Part model, mm, in its own coordinate system. A direction names the side the tool comes from. Round coordinates to 2 decimals unless told otherwise and drop trailing zeros. Write each loop counter-clockwise with the first axis right and the second up, starting at its lowest first coordinate (ties: lowest second). Pieces come first, ordered by that corner, then holes. Notation, with made-up numbers: (14.5, -8.75) -> (34.5, -8.75) arc R22 ccw to (34.5, 12.25) -> close; hole circle Ø6 at (45, 28). An arc over 180 degrees is marked (long way). Use CSV: the item, a comma, the result in double quotes. Start each with the question number.
(1) Saw through at A-A (y = 13.5). Give the cut face in (x, z) (3 decimals).
(2) Saw through at D-D (y = 4.5). Give the cut face in (x, z), plus the area to 3 significant figures.
(3) Saw through at B-B (x = 0.25). Count the separate pieces of the cut face and the enclosed holes in it, plus the area to 3 significant figures.
(4) Saw through at C-C (z = 11.5). Give the cut face in (x, y) (3 decimals), plus the area to 3 significant figures.
(5) Probe line 1 (X direction, y = 1, z = 13) (3 decimals); line 2 (X direction, y = 9.5, z = 9.25); line 3 (Y direction, x = 7, z = 2.75). List the from-to ranges inside material, lowest first. Write a range as [from, to].
(6) Drop flat-ended pins along their axis: pin 1 (0.9 mm diameter, centred on y = -0.5, z = 16.5, fed in from -X); pin 2 (0.5 mm diameter, centred on y = 2.5, z = -0.5, fed in from +X); pin 3 (1.2 mm diameter, centred on x = 1, y = -0.5, fed in from -Z); pin 4 (9 mm diameter, centred on y = 10.5, z = 15.5, fed in from -X). Give the stop position or say it passes through.
(7) Which spindle directions (+Z, -Z, +X, -X, +Y, -Y) get a long thin tool onto all of the face, cutting with end or side? Do faces 5 (the flat face through (-2.315, 11, 1)), 6 (the flat face through (-2.86, -0.5, 16.7)), 7 (the flat face through (-2.315, 1, 11)), 8 (the flat face through (-5.92, 9, 9)), 9 (the flat face through (0, 16.18, -0.5)). Say none if no direction does.
(8) Two-plate mould, pull along Y, no slides. Class faces 1 (the flat face through (0, 2.1, -0.5)), 2 (the flat face through (0, 17.26, -0.5)), 3 (the flat face through (0, -0.5, 2.1)), 4 (the flat face through (0, 7.33, 1)): released by +Y, released by -Y, zero draft, split by the parting line, or undercut.
```python
from build123d import *

# Parameters (mm, degrees)
BOSS_EXTRUDE2_DEPTH     = 7.5
CAVITY_START            = 2
SKETCH3_W               = 5.92
SKETCH3_H               = 9.5
CAVITY_DEPTH            = 23.259018941
SLOT_CUT_REACH          = 26.259
SQUARE_START            = -2
SKETCH8_W               = 2.315
SKETCH8_H               = 6.67
SQUARE_SLOT_DEPTH       = 2
BOSS_EXTRUDE3_DEPTH     = 0.8
SKETCH9_W               = 2.86
SKETCH9_H               = 1.08
SQUARE_RAILS_DEPTH      = 1.08
HALF_START              = 5.92
HALF_MIRROR_DEPTH       = 1.58
HALF_MIRROR_2_OUTLINE_W = 6
HALF_MIRROR_2_OUTLINE_H = 2
HALF_MIRROR_2_DEPTH     = 5.92
HALF_START_2            = 2.315
HALF_MIRROR_3_OUTLINE_W = 6.67
HALF_MIRROR_3_OUTLINE_H = 2
HALF_MIRROR_3_DEPTH     = 3.605
HALF_MIRROR_4_OUTLINE_W = 1.08
HALF_MIRROR_4_OUTLINE_H = 1.08
HALF_MIRROR_4_DEPTH     = 2.86
FULL_START              = -7.5
FULL_MIRROR_OUTLINE_W   = 2
FULL_MIRROR_OUTLINE_H   = 6
FULL_MIRROR_DEPTH       = 15
FULL_MIRROR_2_DEPTH     = 1.58
FULL_START_2            = 5.92
FULL_MIRROR_3_DEPTH     = 1.58
FULL_START_3            = -5.92
FULL_MIRROR_4_OUTLINE_W = 2
FULL_MIRROR_4_OUTLINE_H = 6.67
FULL_MIRROR_4_DEPTH     = 3.605
FULL_START_4            = 2.315
FULL_MIRROR_5_OUTLINE_W = 2
FULL_MIRROR_5_OUTLINE_H = 6.67
FULL_MIRROR_5_DEPTH     = 3.605
FULL_START_5            = -2.86
FULL_MIRROR_6_OUTLINE_W = 1.08
FULL_MIRROR_6_OUTLINE_H = 1.08
FULL_MIRROR_6_DEPTH     = 5.72


# Read off the part's stored shape, not the designer's step: Half mirror, Full mirror
with BuildPart() as part:
    # Sketch2 → Boss-Extrude2 (new body)
    with BuildSketch(Plane(origin=(0, 0, 0), x_dir=(0, 0, -1), z_dir=(1, 0, 0))):
        Polygon((-11.5, 11.5), (-3, 20), (0, 20), (0, 0), align=None)
    extrude(amount=-BOSS_EXTRUDE2_DEPTH)

    # Sketch3 → Cavity (cut, through all)
    with BuildSketch(Plane(origin=(0, 0, 0), x_dir=(1, 0, 0), z_dir=(0, 1, 0)).offset(CAVITY_START)):
        with Locations((-2.96, -6.75)):
            Rectangle(SKETCH3_W, SKETCH3_H)
    extrude(amount=CAVITY_DEPTH, mode=Mode.SUBTRACT)

    # Sketch4 → Slot cut (cut, up to next)
    with BuildSketch(Plane.XY, mode=Mode.PRIVATE) as slot_cut_sk1:
        with BuildLine():
            Line((0, 7.33), (-0.015, 7.33))
            ThreePointArc((-0.015, 7.33), (-1.641345597, 8.003654403), (-2.315, 9.63))
            Line((-2.315, 9.63), (-2.315, 11.7))
            ThreePointArc((-2.315, 11.7), (-1.641345597, 13.326345597), (-0.015, 14))
            Line((-0.015, 14), (0, 14))
            Line((0, 14), (0, 7.33))
        make_face()
    slot_cut_tool1 = extrude(slot_cut_sk1.sketch, amount=SLOT_CUT_REACH, mode=Mode.PRIVATE) & part.part
    add(slot_cut_tool1.solids().sort_by_distance((-1.046523, 10.665, 0))[0], mode=Mode.SUBTRACT)

    # Sketch8 → Square slot (cut)
    with BuildSketch(Plane(origin=(0, 0, 0), x_dir=(-1, 0, 0), z_dir=(0, 0, -1)).offset(SQUARE_START)):
        with Locations((1.1575, 10.665)):
            Rectangle(SKETCH8_W, SKETCH8_H)
    extrude(amount=SQUARE_SLOT_DEPTH, mode=Mode.SUBTRACT)

    # Sketch6 → Boss-Extrude3 (add)
    with BuildSketch(Plane(origin=(0, 0, 0), x_dir=(-1, 0, 0), z_dir=(0, 0, -1))):
        with BuildLine():
            Line((0, 3.18), (2.33, 3.18))
            ThreePointArc((2.33, 3.18), (2.704766594, 3.024766594), (2.86, 2.65))
            Line((2.86, 2.65), (2.86, 2.63))
            ThreePointArc((2.86, 2.63), (2.704766594, 2.255233406), (2.33, 2.1))
            Line((2.33, 2.1), (0, 2.1))
            Line((0, 2.1), (0, 3.18))
        make_face()
        with BuildLine():
            Line((0, 17.26), (2.33, 17.26))
            ThreePointArc((2.33, 17.26), (2.704766594, 17.104766594), (2.86, 16.73))
            Line((2.86, 16.73), (2.86, 16.71))
            ThreePointArc((2.86, 16.71), (2.704766594, 16.335233406), (2.33, 16.18))
            Line((2.33, 16.18), (0, 16.18))
            Line((0, 16.18), (0, 17.26))
        make_face()
    extrude(amount=BOSS_EXTRUDE3_DEPTH)

    # Sketch9 → Square rails (add)
    with BuildSketch(Plane(origin=(0, 0, 0), x_dir=(-1, 0, 0), z_dir=(0, 0, -1))):
        with Locations((1.43, 16.72)):
            Rectangle(SKETCH9_W, SKETCH9_H)
        with Locations((1.43, 2.64)):
            Rectangle(SKETCH9_W, SKETCH9_H)
    extrude(amount=SQUARE_RAILS_DEPTH)



with BuildPart() as body_2:
    # Half mirror outline → Half mirror (new body)
    with BuildSketch(Plane.YZ.offset(HALF_START)):
        Polygon((0, 0), (20, 0), (20, 3), (11.5, 11.5), align=None)
    extrude(amount=HALF_MIRROR_DEPTH)


with BuildPart() as part_1:
    add(part.part)

    add(body_2.part)  # Half mirror 2 merges body 2
    # Half mirror 2 outline → Half mirror 2 (add)
    with BuildSketch(Plane.YZ):
        Polygon((2, 2), (0, 0), (7.33, 0), (7.33, 2), align=None)
        with Locations((17, 1)):
            Rectangle(HALF_MIRROR_2_OUTLINE_W, HALF_MIRROR_2_OUTLINE_H)
    extrude(amount=HALF_MIRROR_2_DEPTH)

    # Half mirror 3 outline → Half mirror 3 (add)
    with BuildSketch(Plane.YZ.offset(HALF_START_2)):
        with Locations((10.665, 1)):
            Rectangle(HALF_MIRROR_3_OUTLINE_W, HALF_MIRROR_3_OUTLINE_H)
    extrude(amount=HALF_MIRROR_3_DEPTH)

    # Half mirror 4 outline → Half mirror 4 (add)
    with BuildSketch(Plane.YZ):
        with Locations((2.64, -0.54)):
            Rectangle(HALF_MIRROR_4_OUTLINE_W, HALF_MIRROR_4_OUTLINE_H)
        with Locations((16.72, -0.54)):
            Rectangle(HALF_MIRROR_4_OUTLINE_W, HALF_MIRROR_4_OUTLINE_H)
    extrude(amount=HALF_MIRROR_4_DEPTH)

    # Full mirror outline → Full mirror (add)
    with BuildSketch(Plane.YZ.offset(FULL_START)):
        Polygon((0, 7.33), (0, 0), (2, 2), (2, 7.33), align=None)
        with Locations((1, 17)):
            Rectangle(FULL_MIRROR_OUTLINE_W, FULL_MIRROR_OUTLINE_H)
    extrude(amount=FULL_MIRROR_DEPTH)

    # Full mirror 2 outline → Full mirror 2 (add)
    with BuildSketch(Plane.YZ.offset(FULL_START)):
        Polygon((2, 7.33), (2, 2), (11.5, 11.5), (3, 20), (2, 20), (2, 14), (0, 14), (0, 7.33), align=None)
    extrude(amount=FULL_MIRROR_2_DEPTH)

    # Full mirror 3 outline → Full mirror 3 (add)
    with BuildSketch(Plane.YZ.offset(FULL_START_2)):
        Polygon((2, 7.33), (2, 2), (11.5, 11.5), (3, 20), (2, 20), (2, 14), (0, 14), (0, 7.33), align=None)
    extrude(amount=FULL_MIRROR_3_DEPTH)

    # Full mirror 4 outline → Full mirror 4 (add)
    with BuildSketch(Plane.YZ.offset(FULL_START_3)):
        with Locations((1, 10.665)):
            Rectangle(FULL_MIRROR_4_OUTLINE_W, FULL_MIRROR_4_OUTLINE_H)
    extrude(amount=FULL_MIRROR_4_DEPTH)

    # Full mirror 5 outline → Full mirror 5 (add)
    with BuildSketch(Plane.YZ.offset(FULL_START_4)):
        with Locations((1, 10.665)):
            Rectangle(FULL_MIRROR_5_OUTLINE_W, FULL_MIRROR_5_OUTLINE_H)
    extrude(amount=FULL_MIRROR_5_DEPTH)

    # Full mirror 6 outline → Full mirror 6 (add)
    with BuildSketch(Plane.YZ.offset(FULL_START_5)):
        with Locations((-0.54, 2.64)):
            Rectangle(FULL_MIRROR_6_OUTLINE_W, FULL_MIRROR_6_OUTLINE_H)
        with Locations((-0.54, 16.72)):
            Rectangle(FULL_MIRROR_6_OUTLINE_W, FULL_MIRROR_6_OUTLINE_H)
    extrude(amount=FULL_MIRROR_6_DEPTH)


solid = part_1.part
```
Answers:
1,outline,"(-7.5, 0) -> (-2.315, 0) -> (-2.315, 2) -> (-5.92, 2) -> (-5.92, 9.5) -> (-7.5, 9.5) -> close; (2.315, 0) -> (7.5, 0) -> (7.5, 9.5) -> (5.92, 9.5) -> (5.92, 2) -> (2.315, 2) -> close"
2,outline,"(-7.5, 0) -> (7.5, 0) -> (7.5, 18.5) -> (5.92, 18.5) -> (5.92, 2) -> (-5.92, 2) -> (-5.92, 18.5) -> (-7.5, 18.5) -> close"
2,area,"82.1 mm²"
3,separate pieces,"3"
3,enclosed holes,"0"
3,area,"54.0 mm²"
4,outline,"(-7.5, 0) -> (-2.315, 0) -> (-2.315, 2) -> (-5.92, 2) -> (-5.92, 11.5) -> (-7.5, 11.5) -> close; (2.315, 0) -> (7.5, 0) -> (7.5, 11.5) -> (5.92, 11.5) -> (5.92, 2) -> (2.315, 2) -> close"
4,area,"50.8 mm²"
5,line 1,"x = [-7.5, -2.315], [2.315, 7.5]"
5,line 2,"x = [-7.5, -5.92], [5.92, 7.5]"
5,line 3,"y = [0, 20]"
6,pin 1,"stops at x = -2.86"
6,pin 2,"stops at x = 2.86"
6,pin 3,"stops at z = 0"
6,pin 4,"stops at x = -7.5"
7,face 5,"+Z, -Z"
7,face 6,"+Z, -Z, -X, -Y"
7,face 7,"+Y, -Y"
7,face 8,"+Z, +Y"
7,face 9,"-Z, +X, -X"
8,face 1,"released by -Y"
8,face 2,"released by +Y"
8,face 3,"zero draft"
8,face 4,"undercut"
